from build123d import *

# Parameters (mm, degrees)
BASE_EXTRUDE_DEPTH = 142.875
CUT_EXTRUDE1_REACH = 236.95
SKETCH2_R          = 8.382
CUT_EXTRUDE2_REACH = 57.372
SKETCH3_R          = 6.731


with BuildPart() as part:
    # Sketch1 → Base-Extrude (new body)
    with BuildSketch(Plane(origin=(0, 0, 0), x_dir=(0, 0, -1), z_dir=(1, 0, 0))):
        with BuildLine():
            Line((0, 0), (-222.25, 0))
            ThreePointArc((-222.25, 0), (-231.230256121, -3.719743879), (-234.95, -12.7))
            Line((-234.95, -12.7), (-234.95, -55.372))
            Line((-234.95, -55.372), (-228.6, -55.372))
            Line((-228.6, -55.372), (-228.6, -12.7))
            ThreePointArc((-228.6, -12.7), (-226.740128061, -8.209871939), (-222.25, -6.35))
            Line((-222.25, -6.35), (0, -6.35))
            Line((0, -6.35), (0, 0))
        make_face()
    extrude(amount=-BASE_EXTRUDE_DEPTH)

    # Sketch2 → Cut-Extrude1 (cut, up to next)
    with BuildSketch(Plane.XY.offset(234.95), mode=Mode.PRIVATE) as cut_extrude1_sk1:
        with Locations((-120.65, -26.9875)):
            Circle(SKETCH2_R)
    cut_extrude1_tool1 = extrude(cut_extrude1_sk1.sketch, amount=-CUT_EXTRUDE1_REACH, mode=Mode.PRIVATE) & part.part
    add(cut_extrude1_tool1.solids().sort_by_distance((-120.65, -26.9875, 234.95))[0], mode=Mode.SUBTRACT)
    # Sketch2 → Cut-Extrude1 (cut, up to next)
    with BuildSketch(Plane.XY.offset(234.95), mode=Mode.PRIVATE) as cut_extrude1_sk2:
        with Locations((-22.225, -26.9875)):
            Circle(SKETCH2_R)
    cut_extrude1_tool2 = extrude(cut_extrude1_sk2.sketch, amount=-CUT_EXTRUDE1_REACH, mode=Mode.PRIVATE) & part.part
    add(cut_extrude1_tool2.solids().sort_by_distance((-22.225, -26.9875, 234.95))[0], mode=Mode.SUBTRACT)

    # Sketch3 → Cut-Extrude2 (cut, up to next)
    with BuildSketch(Plane(origin=(0, 0, 0), x_dir=(-1, 0, 0), z_dir=(0, 1, 0)), mode=Mode.PRIVATE) as cut_extrude2_sk1:
        with Locations((31.75, 95.25)):
            Circle(SKETCH3_R)
    cut_extrude2_tool1 = extrude(cut_extrude2_sk1.sketch, amount=-CUT_EXTRUDE2_REACH, mode=Mode.PRIVATE) & part.part
    add(cut_extrude2_tool1.solids().sort_by_distance((-31.75, 0, 95.25))[0], mode=Mode.SUBTRACT)
    # Sketch3 → Cut-Extrude2 (cut, up to next)
    with BuildSketch(Plane(origin=(0, 0, 0), x_dir=(-1, 0, 0), z_dir=(0, 1, 0)), mode=Mode.PRIVATE) as cut_extrude2_sk2:
        with Locations((31.75, 25.4)):
            Circle(SKETCH3_R)
    cut_extrude2_tool2 = extrude(cut_extrude2_sk2.sketch, amount=-CUT_EXTRUDE2_REACH, mode=Mode.PRIVATE) & part.part
    add(cut_extrude2_tool2.solids().sort_by_distance((-31.75, 0, 25.4))[0], mode=Mode.SUBTRACT)
    # Sketch3 → Cut-Extrude2 (cut, up to next)
    with BuildSketch(Plane(origin=(0, 0, 0), x_dir=(-1, 0, 0), z_dir=(0, 1, 0)), mode=Mode.PRIVATE) as cut_extrude2_sk3:
        Polygon((142.875, 215.9), (50.8, 0), (142.875, 0), align=None)
    cut_extrude2_tool3 = extrude(cut_extrude2_sk3.sketch, amount=-CUT_EXTRUDE2_REACH, mode=Mode.PRIVATE) & part.part
    add(cut_extrude2_tool3.solids().sort_by_distance((-112.183333, 0, 71.966667))[0], mode=Mode.SUBTRACT)


solid = part.part
For this review, take the finished solid that the model builds, in its own axes (mm). A direction names the side the tool comes from. Round coordinates to 2 decimals unless told otherwise and drop trailing zeros. Write each loop counter-clockwise with the first axis right and the second up, starting at its lowest first coordinate (ties: lowest second). Pieces come first, ordered by that corner, then holes. Notation, with made-up numbers: M -9,38 L -4,38 A15 cw -4,52 Z; hole C -15,-20 d1. An arc over 180 degrees is marked long. Write item = value, one per line. Start each with the question number.
(1) We need section C-C (x = -47.5). Give the boundary of the cut face in (y, z), then the cut area to 3 significant figures.
(2) We need section D-D (y = -45.5). Give the boundary of the cut face in (x, z) (3 decimals), then the cut area to 3 significant figures.
(3) For faces 1 (the face through (-70, -34, 228.6)), 2 (the face through (-25, -3, 0)), list the 3-axis set-ups (+Z, -Z, +X, -X, +Y, -Y) from which the entire face can be reached by the end or side of a thin tool; tool diameter is ignored.
(4) The part is to be moulded in two halves that separate along X. For faces 3 (the face through (0, -5, 144)), 4 (the face through (-97.5, -3.1, 109.5)), 5 (the face through (-30.874, -3.131, 101.924)), 6 (the face through (-70, -34, 234.95)), say which applies: +X half, -X half, draft (parallel to the pull), parting line (faces both ways), or undercut.
(5) We need section B-B (z = 25.4). Give the boundary of the cut face in (x, y).
(6) We need section A-A (x = -120.65). Give the boundary of the cut face in (y, z), then the cut area to 3 significant figures.
(7) For line 1 along Z through (x, y) = (-31, -2); line 2 along Y through (x, z) = (-54, 164.5); line 3 along Z through (x, y) = (-80, -36), list the stretches that pass through material, from the lowest coordinate up.
(8) Clearance check with flat-ended pins moving along their axes: pin 1 Ø11 at (x, z) = (-31.75, 95.25) entering from +Y; pin 2 Ø4 at (x, y) = (-116, -9) entering from -Z; pin 3 Ø19.5 at (x, y) = (-120.65, -26.99) entering from -Z; pin 4 Ø1 at (x, z) = (-94, 167.5) entering from -Y. State where each tip first meets the part, or that it passes through.
Results found:
q1.outline = M -55.37,228.6 L -12.7,228.6 A6.35 cw -6.35,222.25 L -6.35,0 L 0,0 L 0,222.25 A12.7 ccw -12.7,234.95 L -55.37,234.95 Z
q1.area = 1,780 mm²
q2.outline = M -142.875,228.6 L 0,228.6 L 0,234.95 L -142.875,234.95 Z
q2.area = 907 mm²
q3.face_1 = -Z, +X, -X, -Y
q3.face_2 = -Z, +X, -X, +Y, -Y
q4.face_3 = +X half
q4.face_4 = -X half
q4.face_5 = undercut
q4.face_6 = draft
q5.outline = M -61.63,-6.35 L -38.48,-6.35 L -38.48,0 L -61.63,0 Z; M -25.02,-6.35 L 0,-6.35 L 0,0 L -25.02,0 Z
q6.outline = M -55.37,228.6 L -35.37,228.6 L -35.37,234.95 L -55.37,234.95 Z; M -18.61,228.6 L -12.7,228.6 A6.35 cw -6.35,222.25 L -6.35,163.79 L 0,163.79 L 0,222.25 A12.7 ccw -12.7,234.95 L -18.61,234.95 Z
q6.area = 631 mm²
q7.line_1 = 0 to 18.71, 32.09 to 88.56, 101.94 to 229.09
q7.line_2 = -6.35 to 0
q7.line_3 = 228.6 to 234.95
q8.pin_1 = through
q8.pin_2 = 225.05
q8.pin_3 = 228.6
q8.pin_4 = -6.35
